The figure shows three views and two pictorial views of one solid part (mm, origin at its lowest corner). Answer the questions. A direction names the side the tool comes from. Give positions to 0.01 mm unless a question says otherwise; leave off trailing zeros. Order: outer loops, then holes, each group sorted by start corner. A loop starts at its lowest first (then second) coordinate and runs counter-clockwise, first axis right, second up. Notation, with made-up numbers: M 7.25,28 L 12.25,28 A17 ccw 12.25,56 Z; hole C -27.75,78 d1. An arc over 180 degrees is marked long. One line per item, written item: value.
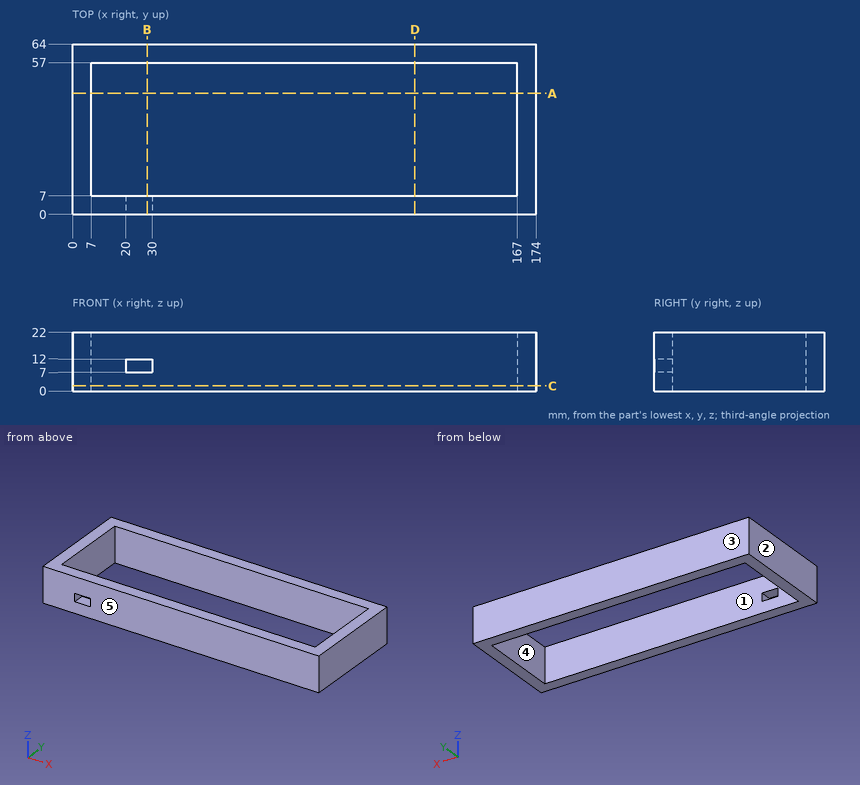
1) Find section B-B, the plane x = 28. Write down the section's boundary in (y, z), plus the area to 3 significant figures.
Reported:
outline: M 0,0 L 7,0 L 7,7 L 0,7 Z; M 0,12 L 7,12 L 7,22 L 0,22 Z; M 57,0 L 64,0 L 64,22 L 57,22 Z
area: 273 mm^2
2) Consider probe 1 along X at (y, z) = (22.5, 3.5); probe 2 along Y at (x, z) = (165, 20); probe 3 along X at (y, z) = (5.5, 11.75). Determine where each line is inside the solid, lowest interval first.
Reported:
probe 1: x = 0 to 7, 167 to 174
probe 2: y = 0 to 7, 57 to 64
probe 3: x = 0 to 20, 30 to 174
3) Find section C-C, the plane z = 2. Write down the section's boundary in (x, y).
Reported:
outline: M 0,0 L 174,0 L 174,64 L 0,64 Z; hole M 7,7 L 167,7 L 167,57 L 7,57 Z
4) Find section D-D, the plane x = 128.5. Write down the section's boundary in (y, z).
Reported:
outline: M 0,0 L 7,0 L 7,22 L 0,22 Z; M 57,0 L 64,0 L 64,22 L 57,22 Z
5) Determine the mould class of the marked faces 1, 2 and 3 for opening direction Y: +Y half, -Y half, draft (parallel to the pull), parting line (faces both ways), or undercut.
Reported:
face 1: undercut
face 2: draft
face 3: +Y half
6) Find section A-A, the plane y = 45.5. Write down the section's boundary in (x, z).
Reported:
outline: M 0,0 L 7,0 L 7,22 L 0,22 Z; M 167,0 L 174,0 L 174,22 L 167,22 Z
7) Which of the six approach directions +Z, -Z, +X, -X, +Y, -Y give full straight-line access (tool end or side, diameter ignored) to the marked faces 4 and 5?
Reported:
face 4: +Z, -Z
face 5: +Z, -Z, +X, -X, -Y
